from build123d import *

# Parameters (mm, degrees)
SKETCH1_R           = 8.001
BOSS_EXTRUDE1_DEPTH = 6.35
SKETCH3_R           = 8.001
BOSS_EXTRUDE2_DEPTH = 12.7
CUT_EXTRUDE1_DEPTH  = 12.7
SKETCH11_R          = 1.905
BOSS_EXTRUDE5_DEPTH = 17.78


with BuildPart() as part:
    # Sketch1 → Boss-Extrude1 (new body)
    with BuildSketch(Plane(origin=(0, 0, 0), x_dir=(1, 0, 0), z_dir=(0, 1, 0))):
        Circle(SKETCH1_R)
    extrude(amount=BOSS_EXTRUDE1_DEPTH)

    # Sketch3 → Boss-Extrude2 (add)
    with BuildSketch(Plane(origin=(0, 0, 0), x_dir=(-1, 0, 0), z_dir=(0, -1, 0))):
        Circle(SKETCH3_R)
    extrude(amount=BOSS_EXTRUDE2_DEPTH)

    # Sketch4 → Cut-Extrude1 (cut)
    with BuildSketch(Plane.XZ.offset(12.7)):
        Polygon((8.54e-07, 2.793990901), (-1.975654462, 4.769648278), (-4.769655316, 1.975649132), (-2.794, -8.246e-06), (-4.769655493, -1.975665446), (-1.97565137, -4.769661323), (0, -2.794), (1.975656347, -4.769656347), (4.769656347, -1.975656347), (2.794, 0), (4.76965137, 1.975661323), (1.975647247, 4.7696572), align=None)
    extrude(amount=-CUT_EXTRUDE1_DEPTH, mode=Mode.SUBTRACT)

    # Sketch11 → Boss-Extrude5 (add)
    with BuildSketch(Plane(origin=(0, 6.35, 0), x_dir=(1, 0, 0), z_dir=(0, 1, 0))):
        Polygon((0, 6.892407514), (-5.969, 3.446203757), (-5.969, -3.446203757), (0, -6.892407514), (5.969, -3.446203757), (5.969, 3.446203757), align=None)
        Circle(SKETCH11_R, mode=Mode.SUBTRACT)
    extrude(amount=BOSS_EXTRUDE5_DEPTH)


solid = part.part
Here's how the part is built. I have some questions about the finished solid (model axes, mm). A direction names the side the tool comes from. Coordinates: 2 decimals unless noted, no trailing zeros. Loops run counter-clockwise (first coordinate to the right, second up) from the corner with the lowest first, then second, coordinate; pieces in that order, holes last. Notation, with made-up numbers: (16.5, 35) -> (42.5, 35) arc R16 cw to (42.5, 49) -> close; hole circle Ø1 at (73.25, 13). An arc over 180 degrees is marked (long way). Use one line per item in the form item = value. Start each with the question number.
(1) Will these pins go through, and if not, where does the flat tip stop? pin 1 (1 mm diameter, centred on y = 3.5, z = -4, fed in from -X); pin 2 (2 mm diameter, centred on y = 16, z = -1.5, fed in from +X); pin 3 (3 mm diameter, centred on y = 14, z = -5, fed in from +X).
(2) If we section it at D-D (y = 14.5): Please give me the cut outline in (x, z) (3 decimals).
(3) If we section it at C-C (x = -5.25): Please give me the cut outline in (y, z).
(4) Please list where these lines run through material, in increasing order: line 1 along X through (y, z) = (13.5, 0) (3 decimals); line 2 along Z through (x, y) = (0, 13.5) (3 decimals); line 3 along Y through (x, z) = (-4.25, 6.5).
(5) If we section it at B-B (z = 6.25): Please give me the cut outline in (x, y), then the cut area to 3 significant figures.
(6) On a 3-axis mill with a long thin cutter (end or side, diameter ignored), from which of +Z, -Z, +X, -X, +Y, -Y can I reach the whole of each face in a straight line? I mean faces 4 (the face through (2.9, 6.35, -5.4)), 5 (the face through (3.392, -6.439, 3.353)), 6 (the face through (5.969, 15, 0)), 7 (the face through (-5.969, 15, 0)). Say none if no direction works.
(7) If we section it at A-A (y = -8): Please give me the cut outline in (x, z).
(8) We'd pull the mould along Z, two halves only. Please class faces 1 (the face through (-1, 24.13, -2)), 2 (the face through (3.768, -6.439, 0.974)), 3 (the face through (-3.026, 15.116, 5.145)): pulls with the +Z half, pulls with the -Z half, needs draft (parallel to the pull), parting line crosses it, or undercut.
Verdict:
q1.pin_1 = -7.19
q1.pin_2 = 5.97
q1.pin_3 = 5.88
q2.outline = (-5.969, -3.446) -> (0, -6.892) -> (5.969, -3.446) -> (5.969, 3.446) -> (0, 6.892) -> (-5.969, 3.446) -> close; hole circle Ø3.81 at (0, 0)
q3.outline = (-12.7, -6.04) -> (6.35, -6.04) -> (6.35, -3.86) -> (24.13, -3.86) -> (24.13, 3.86) -> (6.35, 3.86) -> (6.35, 6.04) -> (-12.7, 6.04) -> close
q4.line_1 = -5.969 to -1.905, 1.905 to 5.969
q4.line_2 = -6.892 to -1.905, 1.905 to 6.892
q4.line_3 = -12.7 to 6.35
q5.outline = (-5, -12.7) -> (5, -12.7) -> (5, 6.35) -> (1.11, 6.35) -> (1.11, 24.13) -> (-1.11, 24.13) -> (-1.11, 6.35) -> (-5, 6.35) -> close
q5.area = 230 mm²
q6.face_4 = +Y
q6.face_5 = -Y
q6.face_6 = +Z, -Z, +X, +Y
q6.face_7 = +Z, -Z, -X, +Y
q7.outline = circle Ø16 at (0, 0); hole (-4.77, -1.98) -> (-1.98, -4.77) -> (0, -2.79) -> (1.98, -4.77) -> (4.77, -1.98) -> (2.79, 0) -> (4.77, 1.98) -> (1.98, 4.77) -> (0, 2.79) -> (-1.98, 4.77) -> (-4.77, 1.98) -> (-2.79, 0) -> close
q8.face_1 = needs draft
q8.face_2 = undercut
q8.face_3 = pulls with the +Z half
